Model file for the job. Use its own axes, mm. A direction names the side the tool comes from. Round coordinates to 2 decimals unless told otherwise and drop trailing zeros. Loops run counter-clockwise (first coordinate to the right, second up) from the corner with the lowest first, then second, coordinate; pieces in that order, holes last. Notation, with made-up numbers: M 2.5,76 L 20.5,76 A6 cw 20.5,80 Z; hole C 13.5,81.5 d9. An arc over 180 degrees is marked long. Answer in a Markdown table with one row per item.
from build123d import *

# Parameters (mm, degrees)
PAD031_DEPTH           = 7.15
CHAMFER003_SIZE        = 1
SKETCH126_R            = 1.8
POCKET033_DEPTH        = 5
SKETCH135_R            = 1.8
POCKET038_DEPTH        = 5
LINEARPATTERN032_COUNT = 1
LINEARPATTERN032_PITCH = 0
LINEARPATTERN033_COUNT = 1
LINEARPATTERN033_PITCH = 0
SKETCH136_R            = 1.8
POCKET039_DEPTH        = 5
SKETCH137_R            = 1.8
POCKET040_DEPTH        = 5


with BuildPart() as part:
    # Sketch127 → Pad031 (new body)
    with BuildSketch(Plane.XY):
        with BuildLine():
            ThreePointArc((4, 42), (1.171573, 40.828427), (0, 38))
            Line((0, 4), (0, 38))
            ThreePointArc((0, 4), (1.171573, 1.171573), (4, 0))
            Line((38, 0), (4, 0))
            ThreePointArc((38, 0), (40.828427, 1.171573), (42, 4))
            Line((42, 38), (42, 4))
            ThreePointArc((42, 38), (40.828427, 40.828427), (38, 42))
            Line((4, 42), (38, 42))
        make_face()
    extrude(amount=PAD031_DEPTH)

    # Chamfer003
    chamfer003_edges = [part.edges().sort_by_distance(p)[0] for p in [
        (1.171573, 1.171573, 0),
        (0, 21, 0),
        (21, 0, 0),
        (40.828427, 1.171573, 0),
        (42, 21, 0),
        (40.828427, 40.828427, 0),
        (21, 42, 0),
        (1.171573, 40.828427, 0),
    ]]
    chamfer(chamfer003_edges, length=CHAMFER003_SIZE)

    # Sketch126 → Pocket033 (cut)
    with BuildSketch(Plane.XZ):
        with Locations((21, 2.6)):
            Circle(SKETCH126_R)
    pocket033 = extrude(amount=-POCKET033_DEPTH, mode=Mode.SUBTRACT)

    # Sketch135 → Pocket038 (cut)
    with BuildSketch(Plane.YZ):
        with Locations((21, 2.6)):
            Circle(SKETCH135_R)
    pocket038 = extrude(amount=POCKET038_DEPTH, mode=Mode.SUBTRACT)

    # LinearPattern032: Pocket033 ×1
    with Locations(*[(i * LINEARPATTERN032_PITCH, 0, 0) for i in range(1, LINEARPATTERN032_COUNT)]):
        add(pocket033, mode=Mode.SUBTRACT)

    # LinearPattern033: Pocket038 ×1
    with Locations(*[(0, i * LINEARPATTERN033_PITCH, 0) for i in range(1, LINEARPATTERN033_COUNT)]):
        add(pocket038, mode=Mode.SUBTRACT)

    # Sketch136 → Pocket039 (cut)
    with BuildSketch(Plane.XZ.offset(-1.5)):
        with Locations((21, 2.6)):
            Circle(SKETCH136_R)
    extrude(amount=-POCKET039_DEPTH, mode=Mode.SUBTRACT)

    # Sketch137 → Pocket040 (cut)
    with BuildSketch(Plane.YZ.offset(1.5)):
        with Locations((21, 2.6)):
            Circle(SKETCH137_R)
    extrude(amount=POCKET040_DEPTH, mode=Mode.SUBTRACT)


solid = part.part
1. Wall check: probe 1 along Z at (x, y) = (21, 4); probe 2 along X at (y, z) = (3.75, 2.6); probe 3 along Y at (x, z) = (5, 2.75). Give the ranges that are in metal, low to high.
Verdict:
| item | result |
|---|---|
| probe 1 | z = 0 to 0.8, 4.4 to 7.15 |
| probe 2 | x = 0.01 to 19.2, 22.8 to 41.99 |
| probe 3 | y = 0 to 19.21, 22.79 to 42 |
2. Mould opens along X. For faces 1 (the conical face through (40.287, 1.662, 0.271)), 2 (the flat face through (6.5, 21, 3)), 3 (the flat face through (21, 6.5, 3)) say: +X half, -X half, draft (parallel to the pull), parting line (faces both ways), or undercut.
Verdict:
| item | result |
|---|---|
| face 1 | +X half |
| face 2 | -X half |
| face 3 | undercut |
3. Saw through at A-A (y = 21). Write the cut outline in (x, z), and give its area (3 significant figures).
Verdict:
| item | result |
|---|---|
| outline | M 0,4.4 L 6.5,4.4 L 6.5,0.8 L 0.2,0.8 L 1,0 L 41,0 L 42,1 L 42,7.15 L 0,7.15 Z |
| area | 276 mm² |
4. Saw through at B-B (z = 2.6). Write the cut outline in (x, y).
Verdict:
| item | result |
|---|---|
| outline | M 0,4 A4 ccw 4,0 L 19.2,0 L 19.2,6.5 L 22.8,6.5 L 22.8,0 L 38,0 A4 ccw 42,4 L 42,38 A4 ccw 38,42 L 4,42 A4 ccw 0,38 L 0,22.8 L 6.5,22.8 L 6.5,19.2 L 0,19.2 Z |
5. Pin check, flat tips, straight feed: pin 1 (1.5 mm diameter, centred on y = 20, z = 4.5, fed in from -X); pin 2 (1.8 mm diameter, centred on x = 20.5, z = 2.5, fed in from -Y); pin 3 (1.1 mm diameter, centred on y = 20.5, z = 2.5, fed in from -X). Stop position of each tip, or through.
Verdict:
| item | result |
|---|---|
| pin 1 | stops at x = 0 |
| pin 2 | stops at y = 6.5 |
| pin 3 | stops at x = 6.5 |
6. Tool access for faces 4 (the cylindrical face through (22.663, 3.204, 1.911)), 5 (the conical face through (40.338, 40.287, 0.271)): list every direction of +Z, -Z, +X, -X, +Y, -Y with a clear straight run to the whole face (end or side of a thin tool).
Verdict:
| item | result |
|---|---|
| face 4 | -Y |
| face 5 | -Z, +X, +Y |
